Source: CAD feature listing. Evaluate the final solid. Frame: model axes, mm. A direction names the side the tool comes from. Give positions to 0.01 mm unless a question says otherwise; leave off trailing zeros. Write each loop counter-clockwise with the first axis right and the second up, starting at its lowest first coordinate (ties: lowest second). Pieces come first, ordered by that corner, then holes. Notation, with made-up numbers: (-31, 20) -> (-14, 20) arc R15 cw to (-14, 29) -> close; hole circle Ø1 at (76, -37.5). An arc over 180 degrees is marked (long way). Use one line per item in the form item = value. Start each with the question number.
(1) Cut plane A-A, the plane x = 0. Output: boundary loops of the cut face in (y, z).
(2) Material intervals for line 1 along Z through (x, y) = (2.5, 1); line 2 along Y through (x, z) = (-3.5, 7.5); line 3 along X through (y, z) = (0.5, 9.25), sorted ascending. Write a range as from..to.
(3) Cut plane D-D, the plane y = -3.75. Output: boundary loops of the cut face in (x, z), and give its area (3 significant figures).
(4) Cut plane B-B, the plane y = 0. Output: boundary loops of the cut face in (x, z), and give its area (3 significant figures).
(5) First-contact query: P1, Ø6, axis at x = 0.5, y = -3, coming from the -Z side; P2, Ø3, axis at x = -2, z = 9, coming from the +Y side; P3, Ø5, axis at x = -3.5, z = 7.5, coming from the +Y side; P4, Ø2, axis at x = 4, z = 11.5, coming from the -Y side. Flat tips, straight axial feed; report the tip coordinate or a pass-through.
(6) Set-up query: faces 1 (the face through (-1.4, 4.5, 4.25)), 2 (the face through (-6, 0, 2)). Return all of +Z, -Z, +X, -X, +Y, -Y with unobstructed straight access to the full face (end or side cutting, diameter ignored); none if empty.
(7) Cut plane C-C, the plane z = 4.5. Output: boundary loops of the cut face in (x, y).
from build123d import *

# Parameters (mm, degrees)
SKETCH1_R               = 4.5
BOSS_EXTRUDE1_DEPTH     = 17
SKETCH1_3_R             = 6
SKETCH1_3_R_2           = 4.5
BOSS_EXTRUDE2_DEPTH     = 4.25
CUT_EXTRUDE1_DEPTH      = 20
CUT_EXTRUDE1_DEPTH_BACK = 20


with BuildPart() as part:
    # Sketch1 → Boss-Extrude1 (new body)
    with BuildSketch(Plane.XY):
        Circle(SKETCH1_R)
    extrude(amount=BOSS_EXTRUDE1_DEPTH)

    # Sketch1<3> → Boss-Extrude2 (add)
    with BuildSketch(Plane.XY):
        Circle(SKETCH1_3_R)
        Circle(SKETCH1_3_R_2, mode=Mode.SUBTRACT)
    extrude(amount=BOSS_EXTRUDE2_DEPTH)

    # Sketch2 → Cut-Extrude1 (cut, two sides: drawn at the far end of the back side and taken through both)
    with BuildSketch(Plane(origin=(0, 0, 0), x_dir=(0, 0, -1), z_dir=(1, 0, 0)).offset(-CUT_EXTRUDE1_DEPTH_BACK)):
        with BuildLine():
            Line((0, 6), (-0.37, 6))
            ThreePointArc((-0.37, 6), (-0.115349001, 3.426659852), (0, 0.843324554))
            Line((0, 0.843324554), (0, 6))
        make_face()
        with BuildLine():
            Line((0, -6), (0, -0.843324554))
            ThreePointArc((0, -0.843324554), (-0.115349001, -3.426659852), (-0.37, -6))
            Line((-0.37, -6), (0, -6))
        make_face()
    extrude(amount=CUT_EXTRUDE1_DEPTH + CUT_EXTRUDE1_DEPTH_BACK, mode=Mode.SUBTRACT)


solid = part.part
Geometry says:
q1.outline = (-6, 0.37) arc R47.88 ccw to (-0.84, 0) -> (0.84, 0) arc R47.88 ccw to (6, 0.37) -> (6, 4.25) -> (4.5, 4.25) -> (4.5, 17) -> (-4.5, 17) -> (-4.5, 4.25) -> (-6, 4.25) -> close
q2.line_1 = 0..17
q2.line_2 = -2.83..2.83
q2.line_3 = -4.47..4.47
q3.outline = (-4.68, 0.14) -> (4.68, 0.14) -> (4.68, 4.25) -> (2.49, 4.25) -> (2.49, 17) -> (-2.49, 17) -> (-2.49, 4.25) -> (-4.68, 4.25) -> close
q3.area = 102 mm^2
q4.outline = (-6, 0) -> (6, 0) -> (6, 4.25) -> (4.5, 4.25) -> (4.5, 17) -> (-4.5, 17) -> (-4.5, 4.25) -> (-6, 4.25) -> close
q4.area = 166 mm^2
q5.P1 = 0
q5.P2 = 4.47
q5.P3 = 4.39
q5.P4 = -3.35
q6.face_1 = +Z
q6.face_2 = +Z, -Z
q7.outline = circle Ø9 at (0, 0)
